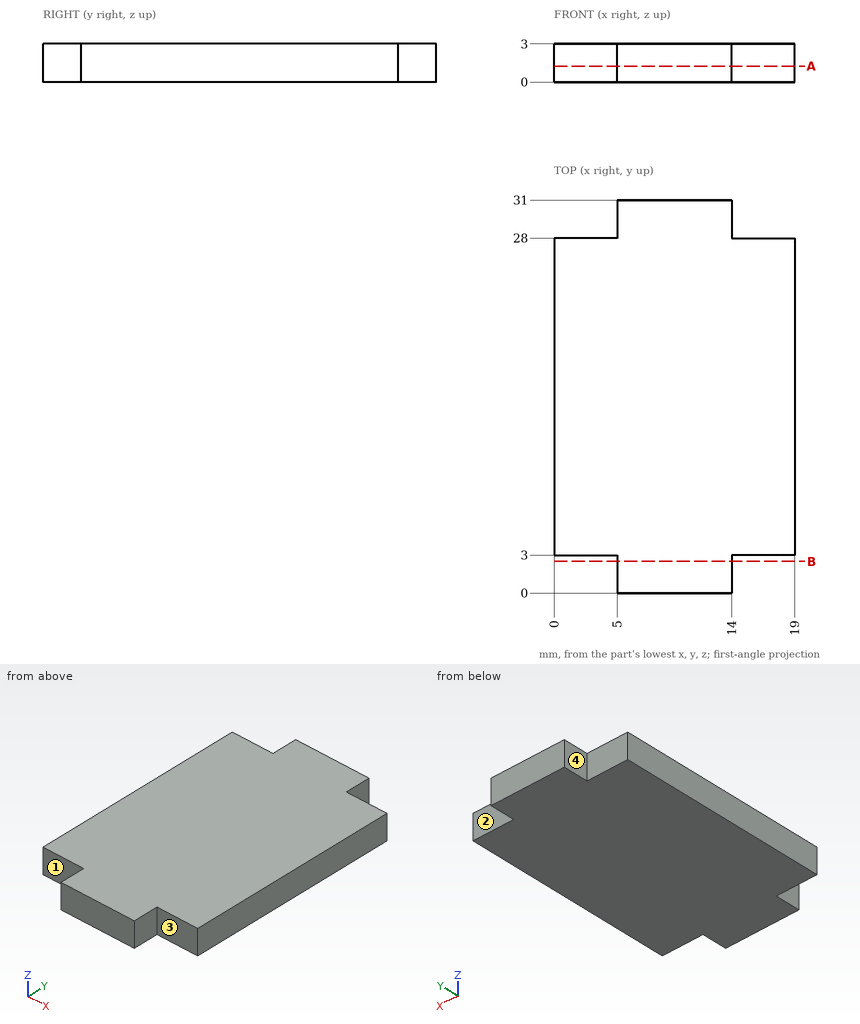
Print and shaded views of the part. All mm, measured from the part's lowest x, y and z. A direction names the side the tool comes from. Coordinates: 2 decimals unless noted, no trailing zeros. Order: outer loops, then holes, each group sorted by start corner. A loop starts at its lowest first (then second) coordinate and runs counter-clockwise, first axis right, second up. Notation, with made-up numbers: (18, 88.25) -> (27, 88.25) arc R23 cw to (27, 118.25) -> close; hole circle Ø9 at (-39, 10). An arc over 180 degrees is marked (long way). Answer as a JSON object with one key per item and string values. Group by question number.
1) Drill centre lines: L1, parallel to Y at x = 3.5, z = 1.55; L2, parallel to X at y = 1, z = 1.25. Where is each one in solid material? Low to high.
2) Which spindle directions (+Z, -Z, +X, -X, +Y, -Y) get a long thin tool onto all of the face, cutting with end or side? Do the marked faces 1, 2, 3 and 4. Say none if no direction does.
3) Cut at B-B, the plane y = 2.5. Write the cut outline in (x, z).
4) Cut at A-A, the plane z = 1.25. Write the cut outline in (x, y), then the cut area to 3 significant figures.
5) Flat gauge pins, fed straight in: pin 1 (1.5 mm diameter, centred on y = 30, z = 1.5, fed in from +X); pin 2 (0.9 mm diameter, centred on x = 16, z = 2, fed in from -Y). Where does each tip first touch, or does it go through?
Check values:
{
 "1": {"L1": "y = 3 to 28", "L2": "x = 5 to 14"},
 "2": {"face 1": "+Z, -Z, -X, -Y", "face 2": "+Z, -Z, +X, +Y", "face 3": "+Z, -Z, +X, -Y", "face 4": "+Z, -Z, -X, +Y"},
 "3": {"outline": "(5, 0) -> (14, 0) -> (14, 3) -> (5, 3) -> close"},
 "4": {"outline": "(0, 3) -> (5, 3) -> (5, 0) -> (14, 0) -> (14, 3) -> (19, 3) -> (19, 28) -> (14, 28) -> (14, 31) -> (5, 31) -> (5, 28) -> (0, 28) -> close", "area": "529 mm²"},
 "5": {"pin 1": "stops at x = 14", "pin 2": "stops at y = 3"}
}
